from build123d import *

# Parameters (mm, degrees)
AUFSATZ_LINEAR_AUSTRAGEN1_DEPTH = 3
SKIZZE4_3_R                     = 10
SKIZZE4_3_R_2                   = 5
AUFSATZ_LINEAR_AUSTRAGEN2_DEPTH = 5
SKIZZE4_4_R                     = 8
SKIZZE4_4_R_2                   = 4
AUFSATZ_LINEAR_AUSTRAGEN3_DEPTH = 4


with BuildPart() as part:
    # Skizze4 → Aufsatz-Linear austragen1 (new body, symmetric)
    with BuildSketch(Plane(origin=(0, 0, 0), x_dir=(1, 0, 0), z_dir=(0, 1, 0))):
        with BuildLine():
            Line((50.32, 7.993597438), (0.4, 9.991996797))
            ThreePointArc((0.4, 9.991996797), (7.211102551, 6.92820323), (10, 0))
            ThreePointArc((10, 0), (7.211102551, -6.92820323), (0.4, -9.991996797))
            Line((0.4, -9.991996797), (50.32, -7.993597438))
            ThreePointArc((50.32, -7.993597438), (42, 0), (50.32, 7.993597438))
        make_face()
    extrude(amount=AUFSATZ_LINEAR_AUSTRAGEN1_DEPTH, both=True)

    # Skizze4_3 → Aufsatz-Linear austragen2 (add, symmetric)
    with BuildSketch(Plane(origin=(0, 0, 0), x_dir=(1, 0, 0), z_dir=(0, 1, 0))):
        with Locations(Location((0, 0, 0), (0, 0, 270))):  # turned: the seam where the file's is
            Circle(SKIZZE4_3_R)
        with Locations(Location((0, 0, 0), (0, 0, 270))):  # turned: the seam where the file's is
            Circle(SKIZZE4_3_R_2, mode=Mode.SUBTRACT)
    extrude(amount=AUFSATZ_LINEAR_AUSTRAGEN2_DEPTH, both=True)

    # Skizze4_4 → Aufsatz-Linear austragen3 (add, symmetric)
    with BuildSketch(Plane(origin=(0, 0, 0), x_dir=(1, 0, 0), z_dir=(0, 1, 0))):
        with Locations(Location((50, 0, 0), (0, 0, 270))):  # turned: the seam where the file's is
            Circle(SKIZZE4_4_R)
        with Locations(Location((50, 0, 0), (0, 0, 270))):  # turned: the seam where the file's is
            Circle(SKIZZE4_4_R_2, mode=Mode.SUBTRACT)
    extrude(amount=AUFSATZ_LINEAR_AUSTRAGEN3_DEPTH, both=True)


solid = part.part
Source: CAD feature listing. Evaluate the final solid. Frame: model axes, mm. A direction names the side the tool comes from. Round coordinates to 2 decimals unless told otherwise and drop trailing zeros. Loops run counter-clockwise (first coordinate to the right, second up) from the corner with the lowest first, then second, coordinate; pieces in that order, holes last. Notation, with made-up numbers: (57.25, -15.75) - (71.25, -15.75) arc R9 ccw to (71.25, -3.75) - close; hole circle Ø1 at (78, 55.5). An arc over 180 degrees is marked (long way). Write item = value, one per line. Start each with the question number.
(1) Pull-direction query (Z, two-part tool) for faces 3 (the face through (-9.76, 0.07, -2.17)), 4 (the face through (54, 4, 2)), 5 (the face through (-4.88, -0.07, -1.08)), 6 (the face through (46.095, -0.056, -0.867)); classes: +Z half, -Z half, draft (parallel to the pull), parting line (faces both ways), or undercut.
(2) Set-up query: faces 1 (the face through (54, -4, 2)), 2 (the face through (5, 5, 2)). Return all of +Z, -Z, +X, -X, +Y, -Y with unobstructed straight access to the full face (end or side cutting, diameter ignored); none if empty.
(3) Pin query (flat end, axial travel): pin 1 (4 mm diameter, centred on x = 36, y = -2.5, fed in from -Z); pin 2 (6.5 mm diameter, centred on x = 50, z = 0, fed in from +Y); pin 3 (2 mm diameter, centred on x = 47, y = -1, fed in from +Z); pin 4 (8 mm diameter, centred on x = 47.5, z = 3, fed in from -Y). Return the tip coordinate at first contact, or that it passes through.
(4) Section query C-C, the plane y = -1.25. Output: boundary loops of the cut face in (x, z), plus the area to 3 significant figures.
(5) Section query A-A, the plane z = 0. Output: boundary loops of the cut face in (x, y).
(6) Section query D-D, the plane z = -6.5. Output: boundary loops of the cut face in (x, y), plus the area to 3 significant figures.
(7) Section query B-B, the plane x = -1.5. Output: boundary loops of the cut face in (y, z).
(8) Ray query, line 1 along X through (y, z) = (2, 0); line 2 along Y through (x, z) = (47, 7.5); line 3 along X through (y, z) = (-2.75, -1.25). Return the intervals inside material, ascending. Write a range as from..to.
Conclusion:
q1.face_3 = parting line
q1.face_4 = draft
q1.face_5 = undercut
q1.face_6 = undercut
q2.face_1 = +Z, -Z, +X, -Y
q2.face_2 = +Z, -Z, +X, -X, +Y
q3.pin_1 = -8.65
q3.pin_2 = through
q3.pin_3 = 8.17
q3.pin_4 = -4
q4.outline = (0.4, -9.99) - (50.32, -7.99) arc R8 ccw to (50.32, 7.99) - (0.4, 9.99) arc R10 ccw (long way) to start; hole circle Ø10 at (0, 0); hole circle Ø8 at (50, 0)
q4.area = 1,030 mm2
q5.outline = (-10, -5) - (-5, -5) - (-5, 5) - (-10, 5) - close; (5, -5) - (10, -5) - (10, -3) - (42, -3) - (42, -4) - (46, -4) - (46, 4) - (42, 4) - (42, 3) - (10, 3) - (10, 5) - (5, 5) - close; (54, -4) - (58, -4) - (58, 4) - (54, 4) - close
q6.outline = (-7.6, -5) - (7.6, -5) - (7.6, -3) - (45.34, -3) - (45.34, -4) - (54.66, -4) - (54.66, 4) - (45.34, 4) - (45.34, 3) - (7.6, 3) - (7.6, 5) - (-7.6, 5) - close
q6.area = 453 mm2
q7.outline = (-5, -9.89) - (5, -9.89) - (5, -4.77) - (-5, -4.77) - close; (-5, 4.77) - (5, 4.77) - (5, 9.89) - (-5, 9.89) - close
q8.line_1 = -10..-5, 5..46, 54..58
q8.line_2 = -3..3
q8.line_3 = -9.92..-4.84, 4.84..46.2, 53.8..57.9
